Work out the finished part from the listing and answer in its coordinate system (mm). Face numbers are marked on the shaded views. Coordinates: 2 decimals unless noted, no trailing zeros. Loops run counter-clockwise (first coordinate to the right, second up) from the corner with the lowest first, then second, coordinate; pieces in that order, holes last. Notation, with made-up numbers: (-16.75, -27.75) -> (-3.75, -27.75) arc R24 ccw to (-3.75, 8.25) -> close; hole circle Ø9 at (73, 66.25). An arc over 180 degrees is marked (long way). One line per question, with ' | ' between items.
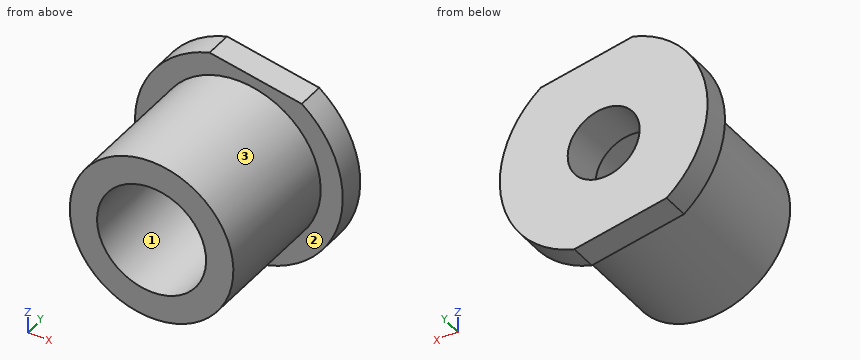
```python
from build123d import *

# Parameters (mm, degrees)
SKETCH2_R          = 3.3
CUT_EXTRUDE1_DEPTH = 21.160636151
SKETCH3_R          = 5
CUT_EXTRUDE2_DEPTH = 11
CUT_EXTRUDE3_DEPTH = 21.160636151


with BuildPart() as part:
    # Sketch1 → Revolve1 (revolve)
    with BuildSketch(Plane.XY, mode=Mode.PRIVATE) as revolve1_sk:
        Polygon((0, 7.5), (-9.525, 7.5), (-9.525, 5), (-7.5, 5), (-7.5, -7.5), (0, -7.5), align=None)
    revolve(revolve1_sk.sketch.rotate(Axis((0, 7.5, 0), (0, -1, 0)), 270), axis=Axis((0, 7.5, 0), (0, -1, 0)))

    # Sketch2 → Cut-Extrude1 (cut, through all)
    with BuildSketch(Plane(origin=(0, 7.5, 0), x_dir=(1, 0, 0), z_dir=(0, 1, 0))):
        with Locations(Location((0, 0, 0), (0, 0, 270))):
            Circle(SKETCH2_R)
    extrude(amount=-CUT_EXTRUDE1_DEPTH, mode=Mode.SUBTRACT)

    # Sketch3 → Cut-Extrude2 (cut)
    with BuildSketch(Plane.XZ.offset(7.5)):
        with Locations(Location((0, 0, 0), (0, 0, 270))):
            Circle(SKETCH3_R)
    extrude(amount=-CUT_EXTRUDE2_DEPTH, mode=Mode.SUBTRACT)

    # Sketch4 → Cut-Extrude3 (cut, through all)
    with BuildSketch(Plane(origin=(0, 7.5, 0), x_dir=(1, 0, 0), z_dir=(0, 1, 0))):
        with BuildLine():
            Line((2.686807128, 9.138199629), (-5.767513864, 7.58033039))
            ThreePointArc((-5.767513864, 7.58033039), (-1.726101863, 9.367294025), (2.686807128, 9.138199629))
        make_face()
        with BuildLine():
            Line((5.767513864, -7.58033039), (-2.686807128, -9.138199629))
            ThreePointArc((-2.686807128, -9.138199629), (1.726101863, -9.367294025), (5.767513864, -7.58033039))
        make_face()
    extrude(amount=-CUT_EXTRUDE3_DEPTH, mode=Mode.SUBTRACT)


solid = part.part
```
1) Find section B-B (x = -0.25). Write down the section's boundary in (y, z).
Check values:
outline: (-7.5, -7.5) -> (5, -7.5) -> (5, -8.6) -> (7.5, -8.6) -> (7.5, -3.29) -> (3.5, -3.29) -> (3.5, -4.99) -> (-7.5, -4.99) -> close; (-7.5, 4.99) -> (3.5, 4.99) -> (3.5, 3.29) -> (7.5, 3.29) -> (7.5, 8.69) -> (5, 8.69) -> (5, 7.5) -> (-7.5, 7.5) -> close
2) Find section A-A (z = 0). Write down the section's boundary in (x, y) (3 decimals).
Check values:
outline: (-9.525, 5) -> (-7.5, 5) -> (-7.5, -7.5) -> (-5, -7.5) -> (-5, 3.5) -> (-3.3, 3.5) -> (-3.3, 7.5) -> (-9.525, 7.5) -> close; (3.3, 3.5) -> (5, 3.5) -> (5, -7.5) -> (7.5, -7.5) -> (7.5, 5) -> (9.525, 5) -> (9.525, 7.5) -> (3.3, 7.5) -> close
3) Find section C-C (y = -0.25). Write down the section's boundary in (x, z).
Check values:
outline: circle Ø15 at (0, 0); hole circle Ø10 at (0, 0)
4) Flat-ended cylindrical pins translate along their axes: pin 1 (6 mm diameter, centred on y = 3, z = -2.5, fed in from -X); pin 2 (5.5 mm diameter, centred on x = 0, z = 0, fed in from -Y); pin 3 (4 mm diameter, centred on x = -1, y = 0.5, fed in from +Z); pin 4 (1.5 mm diameter, centred on y = -4, z = 5.5, fed in from +X). Find the tip coordinate at first contact, or state that the pin passes through.
Check values:
pin 1: stops at x = -9.52 | pin 2: passes through | pin 3: stops at z = 7.5 | pin 4: stops at x = 5.8
5) Find the intervals of material crossed by line 1 along X through (y, z) = (1.25, 0); line 2 along X through (y, z) = (4.5, 0); line 3 along Y through (x, z) = (7.75, -4.5), in increasing order.
Check values:
line 1: x = -7.5 to -5, 5 to 7.5 | line 2: x = -7.5 to -3.3, 3.3 to 7.5 | line 3: y = 5 to 7.5
6) The mould has two halves that part along X. Classify the marked faces 1, 2 and 3: released by +X, released by -X, zero draft, split by the parting line, or undercut.
Check values:
face 1: undercut | face 2: zero draft | face 3: split by the parting line
7) Find section D-D (z = -4.75). Write down the section's boundary in (x, y).
Check values:
outline: (-8.26, 5) -> (-5.8, 5) -> (-5.8, -7.5) -> (-1.56, -7.5) -> (-1.56, 3.5) -> (1.56, 3.5) -> (1.56, -7.5) -> (5.8, -7.5) -> (5.8, 5) -> (8.26, 5) -> (8.26, 7.5) -> (-8.26, 7.5) -> close
